Part print with two shaded views. Sizes in mm from the minimum x, y, z corner. Give positions to 0.01 mm unless a question says otherwise; leave off trailing zeros. Order: outer loops, then holes, each group sorted by start corner. A loop starts at its lowest first (then second) coordinate and runs counter-clockwise, first axis right, second up. Notation, with made-up numbers: (38.25, 74) -> (53.25, 74) arc R24 ccw to (53.25, 98) -> close; hole circle Ø2 at (60, 4.25). An arc over 180 degrees is marked (long way). Write item = value, one per line. Start each with the question number.
Item 1: Band-saw the part on B-B on y = 77. Write the cut outline in (x, z).
Item 2: Flat gauge pins, fed straight in: P1, Ø5, axis at x = 15.5, z = 14, coming from the +Y side; P2, Ø4, axis at x = 10, y = 72.5, coming from the +Z side. Where does each tip first touch, or does it go through?
Item 3: Drill centre lines: line 1 along X through (y, z) = (45, 24.5); line 2 along Z through (x, y) = (43, 76.5). Where is each one in solid material? Low to high.
Item 4: Pull direction X, two halves, no side cores. Call the marked faces 1, 2, 3 and 4: +X half, -X half, draft (parallel to the pull), parting line (faces both ways), or undercut.
Item 5: Band-saw the part on A-A on x = 6.5. Write the cut outline in (y, z), plus the area to 4 significant figures.
Item 6: Band-saw the part on C-C on z = 44.5. Write the cut outline in (x, y).
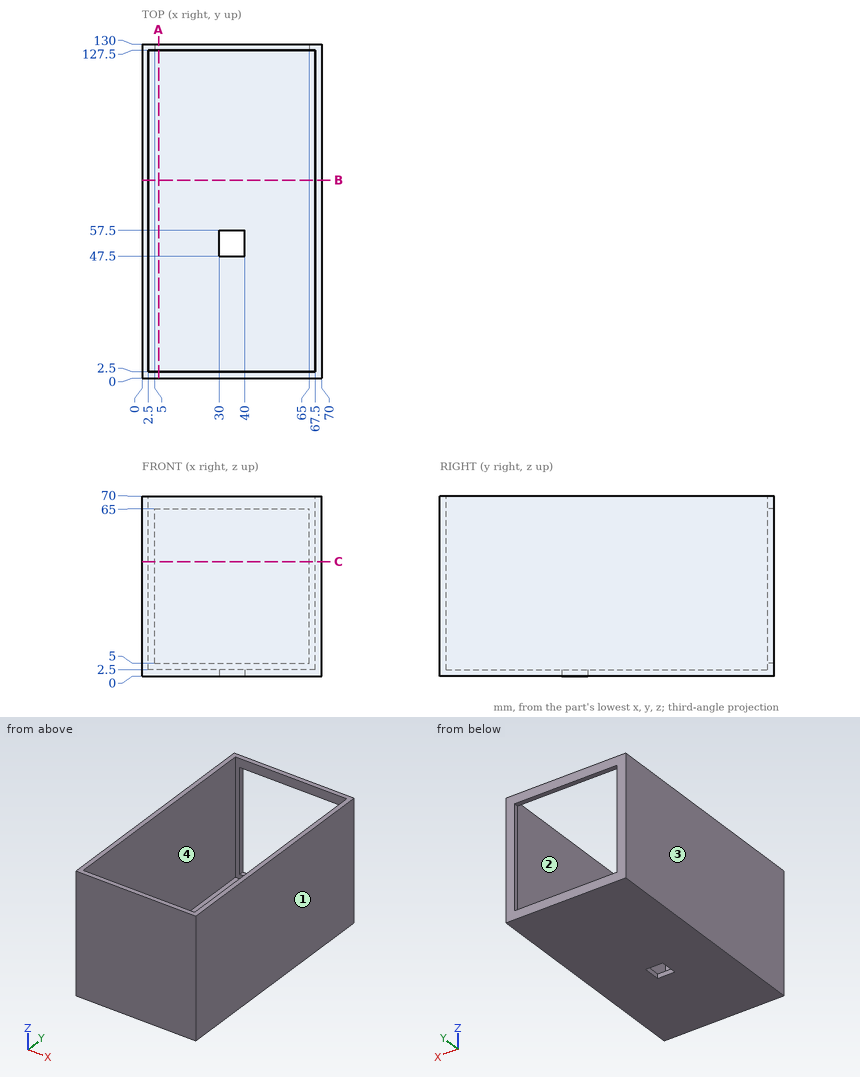
Values found:
q1.outline = (0, 0) -> (70, 0) -> (70, 70) -> (67.5, 70) -> (67.5, 2.5) -> (2.5, 2.5) -> (2.5, 70) -> (0, 70) -> close
q2.P1 = 2.5
q2.P2 = 2.5
q3.line_1 = 0 to 2.5, 67.5 to 70
q3.line_2 = 0 to 2.5
q4.face_1 = +X half
q4.face_2 = undercut
q4.face_3 = -X half
q4.face_4 = undercut
q5.outline = (0, 0) -> (130, 0) -> (130, 5) -> (127.5, 5) -> (127.5, 2.5) -> (2.5, 2.5) -> (2.5, 70) -> (0, 70) -> close; (127.5, 65) -> (130, 65) -> (130, 70) -> (127.5, 70) -> close
q5.area = 512.5 mm^2
q6.outline = (0, 0) -> (70, 0) -> (70, 130) -> (65, 130) -> (65, 127.5) -> (67.5, 127.5) -> (67.5, 2.5) -> (2.5, 2.5) -> (2.5, 127.5) -> (5, 127.5) -> (5, 130) -> (0, 130) -> close
